The listing builds one solid part. Answer for the finished solid, in the listing's coordinates (mm). Face numbers are marked on the shaded views. A direction names the side the tool comes from. Coordinates: 2 decimals unless noted, no trailing zeros. Write each loop counter-clockwise with the first axis right and the second up, starting at its lowest first coordinate (ties: lowest second). Pieces come first, ordered by that corner, then holes. Notation, with made-up numbers: M -34,40.5 L 20,40.5 A22 ccw 20,64.5 Z; hole C -1,-21.5 d11. An arc over 180 degrees is marked long. Answer as CSV lines item,"result". Start each with the question number.
Autodesk Inventor part; units mm, degrees
ref_plane "Work Plane1" through (5, 0, 0) normal (0, 0.5, 0.866) x (1, 0, 0)
ref_plane "YZ Plane" through (0, 0, 0) normal (1, 0, 0) x (0, 1, 0)
ref_plane "XZ Plane" through (0, 0, 0) normal (0, 1, 0) x (-1, 0, 0)
sketch "Sketch1" plane through (0, 0, 0) normal (0, 0, 1) x (1, 0, 0)
  line L0 (-0.6667, 0) -> (10, 0)
  line L1 (10, 0) -> (10, 1.5)
  line L2 (10, 1.5) -> (0, 1.5)
  line L3 (0, 1.5) -> (0, 2.75)
  line L4 (0, 2.75) -> (-3, 2.75)
  line L5 (-3, 2.75) -> (-3, 1.4434)
  line L6 (-3, 1.4434) -> (-1.5, 1.4434)
  line L7 (-1.5, 1.4434) -> (-0.6667, 0)
  line L8 (-25.4, 0) -> (68.4, 0)
  line L9 (0, -1.8) -> (0, 10.8)
  dimension "d3" = 3
  dimension "d4" = 1.5
  dimension "d5" = 60
  dimension "d6" = 3
  dimension "d8" = 2.8868
  dimension "d9" = 5.5
  dimension "d31" = 10
revolve "Body" add sketch "Sketch1" angle 360 about axis through (-0.6667, 0, 0) along (1, 0, 0)
sketch "Sketch2" plane through (-3, 0, 0) normal (-1, 0, 0) x (0, 0, 1)
  circle A0 centre (0, 0) radius 1.4434
  line L0 (0, -8.0829) -> (0, 8.0829)
  line L1 (-8.0829, 0) -> (8.0829, 0)
  line L2 (1.4434, 0) -> (0.7217, -1.25)
  line L3 (0.7217, -1.25) -> (-0.7217, -1.25)
  line L4 (-0.7217, -1.25) -> (-1.4434, 0)
  line L5 (-1.4434, 0) -> (-0.7217, 1.25)
  line L6 (-0.7217, 1.25) -> (0.7217, 1.25)
  line L7 (0.7217, 1.25) -> (1.4434, 0)
extrude "Slot" add sketch "Sketch2" against normal up to next contours L7 A0 | A0 L2 | L6 L0 A0 | A0 L0 L3 | L0 L6 A0 | A0 L3 L0 | L4 A0 | A0 L5
sketch "Sketch3" plane through (-3, 0, 0) normal (-1, 0, 0) x (0, 0, 1)
  circle A0 centre (0, 0) radius 2.75
  line L0 (-0.7217, 1.25) -> (0.7217, 1.25)
  circle A1 centre (0, 0) radius 1.2583
  point P0 (-0.1443, 1.25)
  point P1 (0.1443, 1.25)
  dimension "d23" = 0.2887
extrude "Overcut" cut sketch "Sketch3" against normal blind 1.5 contours A1 L0 | L0 A1
sketch "Sketch4" plane through (0, 0, 0) normal (0, 1, 0) x (-1, 0, 0)
  line L0 (0, 2.75) -> (0, -2.75)
  line L1 (14.4, 0) -> (-2.4, 0)
  circle A0 centre (1.8, 0) radius 0.475
  line L2 (3, 2.75) -> (3, -2.75)
  point P0 (0, 0)
  dimension "d13" = 0.95
  dimension "d14" = 1.2
extrude "Hole" cut sketch "Sketch4" along normal through all both and the other way through all
pattern_circular "Holes" count 3 over 360 about axis through (5, 0, 0) along (1, 0, 0) of "Hole"
chamfer "Chamfer1" distance 0.3 angle 45 1 edges at (-3, -2.75, 0) measured on face at (-1.5904, -2.2485, -1.5833)
thread "Thread"
chamfer "Chamfer2" distance 0.3067 distance2 0.3067 1 edges at (10, -1.5, 0) measured on face at (10, -0.6587, -0.1791)
ref_plane "Work Plane1" through (5, 0, 0) normal (0, 0.5, 0.866) x (1, 0, 0)
equation "\"d3\" = KOH"
equation "\"d4\" = STI"
equation "\"d6\" = GD"
equation "\"d8\" = 1.1547 * SW"
equation "\"d9\" = KOD"
equation "\"d31\" = NLG"
equation "\"d23\" = 0.11547 * SW"
equation "\"d24\" = STI"
equation "\"d13\" = BOR"
equation "\"d14\" = DIST"
equation "\"d17\" = PHH"
equation "\"d32\" = PHH"
equation "\"d19\" = GEL"
equation "\"d21\" = -0.5 * SPD + 0.5 * GD"
equation "\"d22\" = GUL"
equation "\"GD\" = NND"
equation "\"NLG\" = 10"
equation "\"GEL\" = 9"
equation "\"KOD\" = 5.5"
equation "\"KOH\" = 3"
equation "\"GUL\" = 0.61345 * PTC"
equation "\"SW\" = 2.5"
equation "\"STI\" = 1.5"
equation "\"DIST\" = 1.2"
equation "\"BOR\" = 0.95"
equation "\"PHH\" = 0.3"
equation "\"SPD\" = 2.38655"
equation "\"PTC\" = 0.5"
equation "\"THREADDIA\" = 3"
equation "\"TOA\" = 30deg"
equation "\"BDM\" = NND"
equation "\"NND\" = 3"
equation "\"E0\" = 1.155 * SW"
equation "\"GAL\" = 0.61345 * PTC"
equation "\"GD1\" = THREADDIA - 1.2269 * PTC"
properties part number "ANSI B18.3.1M - M3x0,5 x 10" material "Steel, Mild"
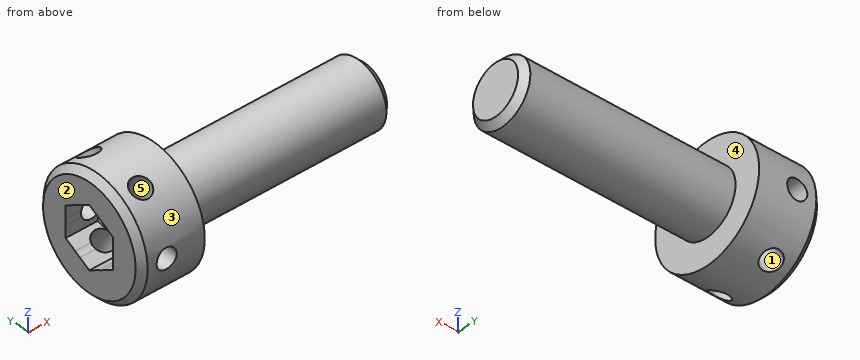
1) Which of the six approach directions +Z, -Z, +X, -X, +Y, -Y give full straight-line access (tool end or side, diameter ignored) to the marked faces 4 and 5?
2) For a pull along Z with two mould halves and no side action, classify the marked faces 1, 2 and 3 as +Z half, -Z half, draft (parallel to the pull), parting line (faces both ways), or undercut.
3) The part is cut by section A-A (x = -1.8). Count the separate pieces of the cut face and the enclosed holes in it, then the cut area to 3 significant figures.
4) Each of these flat-tipped pins is pushed along its axis until it touches: P1, Ø0.5, axis at x = -2, z = 0.5, coming from the -Y side; P2, Ø1.5, axis at x = 8, y = 1.5, coming from the -Z side; P3, Ø0.5, axis at x = -2, z = 0.5, coming from the +Y side. Where does it stop, or does it pass through?
5) The part is cut by section B-B (x = 0.5). Determine the outline of the cut face in (y, z).
6) Find the intervals of material crossed by line 1 (X direction, y = 1.85, z = 0) (3 decimals); line 2 (Z direction, x = -1.8, y = -2.4) (3 decimals); line 3 (Z direction, x = -1.8, y = -2.15) (3 decimals), in increasing order. Write a range as from..to.
Completed:
1,face 4,"+X"
1,face 5,"none"
2,face 1,"undercut"
2,face 2,"draft"
2,face 3,"parting line"
3,separate pieces,"6"
3,enclosed holes,"0"
3,area,"9.87 mm²"
4,P1,"y = -2.73"
4,P2,"z = -1.3"
4,P3,"y = 2.73"
5,outline,"C 0,0 d3"
6,line 1,"-3..-2.275, -1.325..0"
6,line 2,"-1.343..-0.475, 0.475..1.343"
6,line 3,"-1.715..-0.475, 0.475..1.715"
